Answer from the drawing. Dimensions are ordinates in mm from the lowest x, y and z of the part. A direction names the side the tool comes from. Give positions to 0.01 mm unless a question says otherwise; leave off trailing zeros. Write each loop counter-clockwise with the first axis right and the second up, starting at its lowest first coordinate (ties: lowest second). Pieces come first, ordered by that corner, then holes.
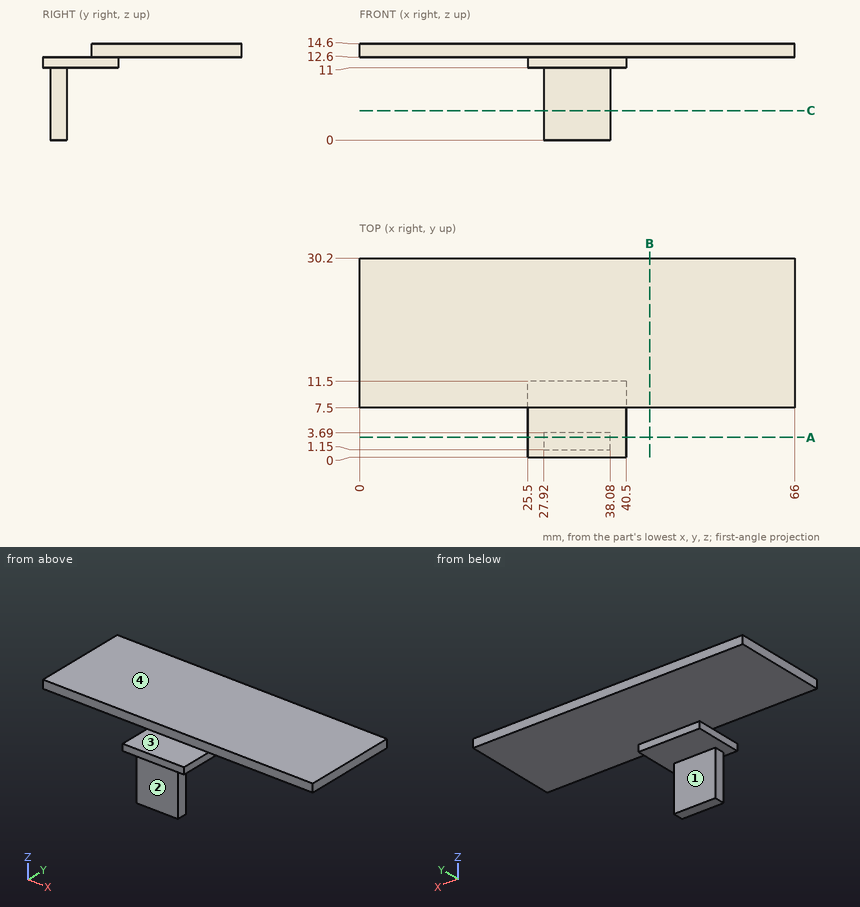
Item 1: Section B-B (x = 44) is taken. Write down the section's boundary in (y, z), and give its area (3 significant figures).
Result set:
outline: (7.5, 12.6) - (30.2, 12.6) - (30.2, 14.6) - (7.5, 14.6) - close
area: 45.4 mm2
Item 2: Find the intervals of material crossed by line 1 along Z through (x, y) = (62, 23.5); line 2 along Y through (x, z) = (61, 13.75); line 3 along Z through (x, y) = (36, 3), in increasing order.
Result set:
line 1: z = 12.6 to 14.6
line 2: y = 7.5 to 30.2
line 3: z = 0 to 12.6
Item 3: Each of these flat-tipped pins is pushed along its axis until it touches: pin 1 Ø6 at (x, y) = (12, 25.5) entering from -Z; pin 2 Ø1.3 at (y, z) = (2, 4.5) entering from +X; pin 3 Ø1.8 at (y, z) = (7, 11.5) entering from -X. Where does it stop, or does it pass through?
Result set:
pin 1: stops at z = 12.6
pin 2: stops at x = 38.08
pin 3: stops at x = 25.5
Item 4: Section C-C (z = 4.5) is taken. Write down the section's boundary in (x, y).
Result set:
outline: (27.92, 1.15) - (38.08, 1.15) - (38.08, 3.69) - (27.92, 3.69) - close
Item 5: Section A-A (y = 3) is taken. Write down the section's boundary in (x, z), and give its area (3 significant figures).
Result set:
outline: (25.5, 11) - (27.92, 11) - (27.92, 0) - (38.08, 0) - (38.08, 11) - (40.5, 11) - (40.5, 12.6) - (25.5, 12.6) - close
area: 136 mm2
Item 6: Which of the six approach directions +Z, -Z, +X, -X, +Y, -Y give full straight-line access (tool end or side, diameter ignored) to the marked faces 1, 2, 3 and 4?
Result set:
face 1: -Z, +X, -X, +Y
face 2: -Z, +X, -X, -Y
face 3: +Z, +X, -X, -Y
face 4: +Z, +X, -X, +Y, -Y
